Verification items for the finished model (mm, model axes). Coordinates: 2 decimals unless noted, no trailing zeros. Order: outer loops, then holes, each group sorted by start corner. A loop starts at its lowest first (then second) coordinate and runs counter-clockwise, first axis right, second up. Notation, with made-up numbers: (25.5, -25.75) -> (29.5, -25.75) arc R34 ccw to (29.5, 8.25) -> close; hole circle Ø5 at (72.5, 77.5). An arc over 180 degrees is marked (long way). Write item = value, one per line. Start each with the question number.
from build123d import *

# Parameters (mm, degrees)
SKETCH1_R           = 1.778
BOSS_EXTRUDE1_DEPTH = 6.35


with BuildPart() as part:
    # Sketch1 → Boss-Extrude1 (new body)
    with BuildSketch(Plane.XZ):
        with BuildLine():
            Line((-48.895, -4.7625), (48.895, -4.7625))
            ThreePointArc((48.895, -4.7625), (53.6575, 0), (48.895, 4.7625))
            Line((48.895, 4.7625), (-48.895, 4.7625))
            ThreePointArc((-48.895, 4.7625), (-53.6575, 0), (-48.895, -4.7625))
        make_face()
        with Locations((48.895, 0)):
            Circle(SKETCH1_R, mode=Mode.SUBTRACT)
        with Locations((39.116, 0)):
            Circle(SKETCH1_R, mode=Mode.SUBTRACT)
        with Locations((29.337, 0)):
            Circle(SKETCH1_R, mode=Mode.SUBTRACT)
        with Locations((19.558, 0)):
            Circle(SKETCH1_R, mode=Mode.SUBTRACT)
        with Locations((9.779, 0)):
            Circle(SKETCH1_R, mode=Mode.SUBTRACT)
        Circle(SKETCH1_R, mode=Mode.SUBTRACT)
        with Locations((-9.779, 0)):
            Circle(SKETCH1_R, mode=Mode.SUBTRACT)
        with Locations((-19.558, 0)):
            Circle(SKETCH1_R, mode=Mode.SUBTRACT)
        with Locations((-29.337, 0)):
            Circle(SKETCH1_R, mode=Mode.SUBTRACT)
        with Locations((-39.116, 0)):
            Circle(SKETCH1_R, mode=Mode.SUBTRACT)
        with Locations((-48.895, 0)):
            Circle(SKETCH1_R, mode=Mode.SUBTRACT)
    extrude(amount=-BOSS_EXTRUDE1_DEPTH)


solid = part.part
Item 1: Thickness scan on line 1 (Z direction, x = 0, y = 3.5); line 2 (Z direction, x = 10.5, y = 3); line 3 (X direction, y = 0.75, z = -4). Record the ranges inside material, lowest first.
Item 2: Section check D-D (x = 19). Record the boundary of the cut face in (y, z).
Item 3: Section check B-B (y = 4). State how many separate pieces and enclosed holes the cut face has, then the cut area to 3 significant figures.
Item 4: Gauge pin test, flat ends, axial feed: P1, Ø3, axis at x = 0, z = 0, coming from the +Y side; P2, Ø1, axis at y = 4, z = -1, coming from the +X side. Record the tip position at first contact, or that the pin passes through.
Item 5: Section check A-A (x = 0). Record the boundary of the cut face in (y, z), then the cut area to 3 significant figures.
Item 6: Mould release check, pull along Z, two halves, no side actions. Record for faces 1 (the cylindrical face through (-47.253, 3.131, -0.681)), 2 (the flat face through (1, 3, 4.762)), 3 (the cylindrical face through (53.656, 3.131, -0.105)): pulls with the +Z half, pulls with the -Z half, needs draft (parallel to the pull), parting line crosses it, or undercut.
Filled sheet:
q1.line_1 = -4.76 to -1.78, 1.78 to 4.76
q1.line_2 = -4.76 to -1.63, 1.63 to 4.76
q1.line_3 = -51.48 to 51.48
q2.outline = (0, -4.76) -> (6.35, -4.76) -> (6.35, -1.69) -> (0, -1.69) -> close; (0, 1.69) -> (6.35, 1.69) -> (6.35, 4.76) -> (0, 4.76) -> close
q3.separate_pieces = 1
q3.enclosed_holes = 11
q3.area = 893 mm^2
q4.P1 = through
q4.P2 = 53.63
q5.outline = (0, -4.76) -> (6.35, -4.76) -> (6.35, -1.78) -> (0, -1.78) -> close; (0, 1.78) -> (6.35, 1.78) -> (6.35, 4.76) -> (0, 4.76) -> close
q5.area = 37.9 mm^2
q6.face_1 = undercut
q6.face_2 = pulls with the +Z half
q6.face_3 = parting line crosses it
